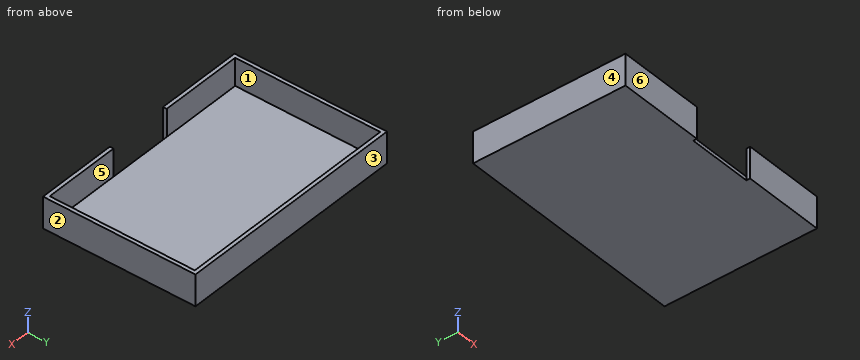
Autodesk Fusion 360 part; units mm, degrees
sketch "Sketch1" plane through (0, 0, 0) normal (0, 0, 1) x (1, 0, 0) in component "stand"
  line L0 (61, -39.5) -> (-61, -39.5)
  line L1 (-61, -39.5) -> (-61, 39.5)
  line L2 (-61, 39.5) -> (61, 39.5)
  line L3 (61, 39.5) -> (61, -39.5)
  line L4 (61, -39.5) -> (-61, 39.5) construction
  line L5 (-61, -39.5) -> (61, 39.5) construction
  line L6 (63, -41.5) -> (-63, -41.5)
  line L7 (-63, -41.5) -> (-63, 41.5)
  line L8 (-63, 41.5) -> (63, 41.5)
  line L9 (63, 41.5) -> (63, -41.5)
  line L10 (-61, 0) -> (-16, 0)
  line L11 (-61, 0) -> (19, 0)
  line L12 (-16, 0) -> (-16, -41.5)
  line L13 (19, 0) -> (19, -41.5)
  line L14 (-61, 39.5) -> (61, 39.5)
  line L15 (-61, 0) -> (19, 0)
  line L16 (-63, 41.5) -> (63, 41.5)
  line L17 (-63, -41.5) -> (-63, 41.5)
  line L18 (-61, 0) -> (-16, 0)
  line L19 (63, 41.5) -> (63, -41.5)
  line L20 (61, 39.5) -> (61, -39.5)
  line L21 (-16, 0) -> (-16, -41.5)
  line L22 (61, -39.5) -> (-61, -39.5)
  line L23 (63, -41.5) -> (-63, -41.5)
  line L24 (-61, -39.5) -> (-61, 39.5)
  line L25 (61, -39.5) -> (-61, 39.5) construction
  line L26 (19, 0) -> (19, -41.5)
  line L27 (-61, -39.5) -> (61, 39.5) construction
  dimension "d1" = 122
  dimension "d2" = 79
  dimension "d3" = -2
  dimension "d4" = 45
  dimension "d5" = 80
  dimension "d10" = -2
  dimension "d11" = 122
  dimension "d12" = 79
  dimension "d13" = 45
  dimension "d14" = 80
extrude "Extrude1" add sketch "Sketch1" along normal blind 17 contours L0 L1 L2 L3 L6 L7 L8 L9 L12 L13 L14 L16 L17 L19 L20 L21 L22 L23 L24 L26 in component "stand"
extrude "Extrude2" add sketch "Sketch1" along normal blind 2 contours L0 L1 L2 L3 L10 L11 L13 L14 L15 L18 L20 L22 L24 L26 | L0 L11 L12 L13 L15 L21 L22 L26 | L0 L1 L10 L11 L12 L15 L18 L21 L22 L24 in component "stand"
component "stand" placed x (1, 0, 0) y (0, 1, 0) z (0, 0, 1) at (0, 0, 0)
Geometry check sheet. Reference: the model listing, model coordinates, mm. Face numbers are marked on the shaded views. A direction names the side the tool comes from. Give positions to 0.01 mm unless a question says otherwise; leave off trailing zeros. Order: outer loops, then holes, each group sorted by start corner. A loop starts at its lowest first (then second) coordinate and runs counter-clockwise, first axis right, second up.
1) Tool access check on the marked faces 5 and 6. Record the directions out of +Z, -Z, +X, -X, +Y, -Y that give a thin tool (end or side, any length) a straight path to the whole face; none if there is none.
Results are:
face 5: +Z
face 6: +Z, -Z, +X, -X, -Y
2) Cross-section at C-C (x = 36). Record the boundary of the cut face in (y, z).
Results are:
outline: (-41.5, 0) - (41.5, 0) - (41.5, 17) - (39.5, 17) - (39.5, 2) - (-39.5, 2) - (-39.5, 17) - (-41.5, 17) - close
3) Cross-section at B-B (y = 9). Record the boundary of the cut face in (x, z), then the cut area to 3 significant figures.
Results are:
outline: (-63, 0) - (63, 0) - (63, 17) - (61, 17) - (61, 2) - (-61, 2) - (-61, 17) - (-63, 17) - close
area: 312 mm2
4) Cross-section at D-D (x = 4). Record the boundary of the cut face in (y, z), then the cut area to 3 significant figures.
Results are:
outline: (-39.5, 0) - (41.5, 0) - (41.5, 17) - (39.5, 17) - (39.5, 2) - (-39.5, 2) - close
area: 192 mm2
5) Cross-section at A-A (z = 15). Record the boundary of the cut face in (x, y), then the cut area to 3 significant figures.
Results are:
outline: (-63, -41.5) - (-16, -41.5) - (-16, -39.5) - (-61, -39.5) - (-61, 39.5) - (61, 39.5) - (61, -39.5) - (19, -39.5) - (19, -41.5) - (63, -41.5) - (63, 41.5) - (-63, 41.5) - close
area: 750 mm2
6) Gauge pin test, flat ends, axial feed: pin 1 (1.5 mm diameter, centred on x = -19.5, y = 22.5, fed in from +Z); pin 2 (1 mm diameter, centred on x = -4.5, z = 1, fed in from -Y). Record the tip position at first contact, or that the pin passes through.
Results are:
pin 1: stops at z = 2
pin 2: stops at y = -39.5
7) Draft check along X on the marked faces 1, 2, 3 and 4. Enter one of: released by +X, released by -X, zero draft, split by the parting line, or undercut.
Results are:
face 1: undercut
face 2: released by +X
face 3: zero draft
face 4: released by -X
8) Material ranges on probe 1 along Y at (x, z) = (-54.5, 9); probe 2 along X at (y, z) = (6.5, 12.75); probe 3 along Y at (x, z) = (1, 9.25), recorded low to high.
Results are:
probe 1: y = -41.5 to -39.5, 39.5 to 41.5
probe 2: x = -63 to -61, 61 to 63
probe 3: y = 39.5 to 41.5
